from build123d import *

# Parameters (mm, degrees)
F1_DEPTH = 30
F3_R     = 13
F3_R_2   = 11
F4_DEPTH = 75


# Not quite as in the source:
# - the program builds the solid bodies; features that only make, move or delete a surface that nothing else refers to are left out


with BuildPart() as f1:
    # F0 (on Top) → F1 (new body)
    with BuildSketch(Plane.XY):
        with BuildLine():
            Line((0, 0), (-15, 0))
            Line((-15, 0), (-60, -71.2145941459))
            ThreePointArc((-60, -71.2145941459), (0, -88.4018294902), (60, -71.2145941459))
            Line((60, -71.2145941459), (15, 0))
            Line((15, 0), (0, 0))
        make_face()
    extrude(amount=F1_DEPTH)

    # F3 (on Front) → F4 (cut)
    with BuildSketch(Plane.XZ):
        with Locations((-34, 15.2476818305)):
            Circle(F3_R)
        with Locations((-34, 15.2476818305)):
            Circle(F3_R_2, mode=Mode.SUBTRACT)
        with Locations((0, 15.1581136116)):
            Circle(F3_R)
        with Locations((0, 15.1581136116)):
            Circle(F3_R_2, mode=Mode.SUBTRACT)
        with Locations((34, 15.0685453927)):
            Circle(F3_R)
        with Locations((34, 15.0685453927)):
            Circle(F3_R_2, mode=Mode.SUBTRACT)
        with Locations((0, 15.1581136116)):
            Circle(F3_R_2)
        with Locations((34, 15.0685453927)):
            Circle(F3_R_2)
        with Locations((-34, 15.2476818305)):
            Circle(F3_R_2)
    extrude(amount=F4_DEPTH, mode=Mode.SUBTRACT)


solid = f1.part
Read the model definition and answer for the solid it produces. Units are mm, in the model's axes. A direction names the side the tool comes from. Coordinates: 2 decimals unless noted, no trailing zeros. Order: outer loops, then holes, each group sorted by start corner. A loop starts at its lowest first (then second) coordinate and runs counter-clockwise, first axis right, second up. Notation, with made-up numbers: (32.25, 86.5) -> (82.25, 86.5) arc R12 ccw to (82.25, 109.5) -> close; hole circle Ø6 at (6.5, -6). An arc over 180 degrees is marked (long way). Answer as a JSON object with one key per item and string values.
1) Consider line 1 along Z through (x, y) = (0, -59); line 2 along X through (y, z) = (-52, 18.25); line 3 along X through (y, z) = (-54.5, 11). Determine where each line is inside the solid, lowest interval first. Write a range as from..to.
Model answer:
{"line 1": "z = 0..2.16, 28.16..30", "line 2": "x = -47.86..-46.65, -21.35..-12.63, 12.63..21.4, 46.6..47.86", "line 3": "x = -49.44..-46.29, -21.71..-12.32, 12.32..21.65, 46.35..49.44"}
2) A cutting plane is placed at D-D, the plane y = -28. Determine the outline of the cut face in (x, z), plus the area to 3 significant figures.
Model answer:
{"outline": "(-32.69, 0) -> (32.69, 0) -> (32.69, 2.13) arc R13 cw to (32.69, 28) -> (32.69, 30) -> (-32.69, 30) -> (-32.69, 28.18) arc R13 cw to (-32.69, 2.31) -> close; hole circle Ø26 at (0, 15.16)", "area": "968 mm²"}
3) A cutting plane is placed at C-C, the plane z = 17.5. Determine the outline of the cut face in (x, y) (1 decimal).
Model answer:
{"outline": "(-60, -71.2) arc R113.3 ccw to (60, -71.2) -> (46.8, -50.3) -> (46.8, -75) -> (21.2, -75) -> (21.2, -9.9) -> (15, 0) -> (12.8, 0) -> (12.8, -75) -> (-12.8, -75) -> (-12.8, 0) -> (-15, 0) -> (-21.2, -9.8) -> (-21.2, -75) -> (-46.8, -75) -> (-46.8, -50.3) -> close"}
4) A cutting plane is placed at A-A, the plane x = 0. Determine the outline of the cut face in (y, z).
Model answer:
{"outline": "(-88.4, 0) -> (0, 0) -> (0, 2.16) -> (-75, 2.16) -> (-75, 28.16) -> (0, 28.16) -> (0, 30) -> (-88.4, 30) -> close"}
5) Each of these flat-tipped pins is pushed along its axis until it touches: pin 1 (2 mm diameter, centred on x = 47.5, z = 25.5, fed in from +Y); pin 2 (4 mm diameter, centred on x = -38, z = 3.5, fed in from +Y); pin 3 (4 mm diameter, centred on x = 2, z = 10, fed in from +Y); pin 4 (12 mm diameter, centred on x = 5.5, z = 20.5, fed in from +Y). Where does it stop, or does it pass through?
Model answer:
{"pin 1": "stops at y = -49.85", "pin 2": "stops at y = -33.7", "pin 3": "stops at y = -75", "pin 4": "stops at y = 0"}
6) The mould has two halves that part along X. Classify faces 3 (the face through (0, 0, 1)), 4 (the face through (-42.185, -43.022, 4.79)), 5 (the face through (21.013, -48.963, 15.64)): released by +X, released by -X, zero draft, split by the parting line, or undercut.
Model answer:
{"face 3": "zero draft", "face 4": "released by -X", "face 5": "undercut"}
7) A cutting plane is placed at B-B, the plane y = -65.5. Determine the outline of the cut face in (x, z), plus the area to 3 significant figures.
Model answer:
{"outline": "(-56.39, 0) -> (56.39, 0) -> (56.39, 30) -> (-56.39, 30) -> close; hole circle Ø26 at (-34, 15.25); hole circle Ø26 at (0, 15.16); hole circle Ø26 at (34, 15.07)", "area": "1,790 mm²"}
8) A tool of negligible diameter and unlimited length cuts with its end or side. For faces 1 (the face through (-1, -53, 30)), 2 (the face through (0, -75, 15)), from which of +Z, -Z, +X, -X, +Y, -Y can it reach the whole face along a straight path? Write none if from no direction.
Model answer:
{"face 1": "+Z, +X, -X, +Y, -Y", "face 2": "+Y"}
